Could you check a few things on this model? Use its own coordinates, in mm. Give positions to 0.01 mm unless a question says otherwise; leave off trailing zeros. Write each question's results on one line, items separated by ' | '. Start each with the question number.
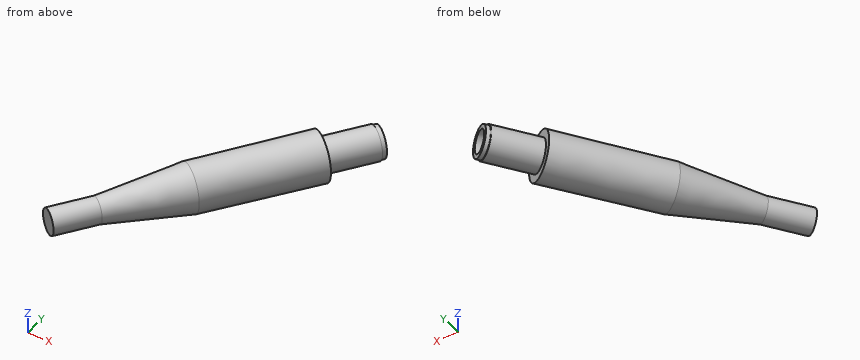
from build123d import *

# Parameters (mm, degrees)
SKETCH2_OUTSIDE_W  = 81.185
SKETCH2_OUTSIDE_H  = 67.044
SKETCH2_OUTSIDE_R  = 3.495
CUT_EXTRUDE1_DEPTH = 1


with BuildPart() as part:
    # Sketch1 → Revolve1 (revolve)
    with BuildSketch(Plane(origin=(96.031948768, 24.259878967, -114.32637478), x_dir=(0.579754018, 0.814791555, 0), z_dir=(0, 0, -1))):
        Polygon((-201.145317806, 47.619722085), (-136.905317806, 47.619722085), (-136.905317806, 47.980853052), (-145.145317806, 47.980853052), (-145.145317806, 50.169722085), (-132.905317806, 50.169722085), (-132.905317806, 51.314722085), (-145.145317806, 51.314722085), (-145.145317806, 53.039722085), (-172.145317806, 52.884722085), (-191.145317806, 50.459722085), (-201.145317806, 50.459722085), align=None)
    revolve(axis=Axis((18.217289915, -167.239352557, -114.32637478), (0.579754018, 0.814791555, 0)))

    # Sketch2 outside → Cut-Extrude1 (cut)
    with BuildSketch(Plane(origin=(-33.314790755, -46.820909057, 0), x_dir=(0.663885278, -0.472378678, -0.579754018), z_dir=(0.579754018, 0.814791555, 0))):
        with Locations((157.4895, 28.254)):
            Rectangle(SKETCH2_OUTSIDE_W, SKETCH2_OUTSIDE_H)
        with Locations((157.375670059, 28.335096914)):
            Circle(SKETCH2_OUTSIDE_R, mode=Mode.SUBTRACT)
    extrude(amount=-CUT_EXTRUDE1_DEPTH, mode=Mode.SUBTRACT)


solid = part.part
Q1. Please list where these lines run through material, in increasing order: line 1 (X direction, y = -116, z = -113); line 2 (X direction, y = -116, z = -115.25); line 3 (Z direction, x = 50.5, y = -119). Write a range as [from, to].
Q2. If we section it at A-A (y = -116.5): Count the separate pieces of the cut face and the enclosed holes in it, plus the area to 3 significant figures.
Q3. I'm going to push flat-ended pins straight in: P1, Ø1, axis at x = 40.5, z = -111.5, coming from the -Y side; P2, Ø3, axis at y = -121, z = -118.5, coming from the -X side; P3, Ø1.5, axis at x = 45, y = -123.5, coming from the +Z side. Where does each tip first touch, or does it pass through?
Determined:
1) line 1: x = [50.44, 52], [57.35, 58.91] | line 2: x = [50.29, 51.76], [57.59, 59.07] | line 3: z = [-117.63, -116.26], [-112.39, -111.03]
2) separate pieces: 2 | enclosed holes: 1 | area: 28.1 mm²
3) P1: stops at y = -144.48 | P2: stops at x = 44.94 | P3: stops at z = -109.71
